CAD build for the part. Positions are in the model's coordinates, mm. A direction names the side the tool comes from. Round coordinates to 2 decimals unless told otherwise and drop trailing zeros. Order: outer loops, then holes, each group sorted by start corner. A loop starts at its lowest first (then second) coordinate and runs counter-clockwise, first axis right, second up. Notation, with made-up numbers: M -30.5,-10 L -0.5,-10 A13 ccw -0.5,8 Z; hole C 69,15 d4. An arc over 180 degrees is marked long. Answer as a JSON object with one key per item and string values. Group by question number.
```python
from build123d import *

# Parameters (mm, degrees)
EXTRUDE_3_DEPTH                 = 15
EXTRUDE_2_DEPTH                 = 1
SKETCH_4_R                      = 5.85
CUT_EXTRUDE_1_DEPTH             = 2
SKIZZE1_W                       = 11.487069154
SKIZZE1_H                       = 62.431572876
SCHNITT_LINEAR_AUSTRAGEN1_DEPTH = 0.5
SKIZZE2_W                       = 1.5
SKIZZE2_H                       = 1.5
AUFSATZ_LINEAR_AUSTRAGEN1_DEPTH = 1.5


with BuildPart() as part:
    # Эскиз1 → Вытянуть-Тонкостенный3 (new body)
    with BuildSketch(Plane.XY):
        Polygon((-21.213203436, -45), (-21.213203436, 45), (0, 66.213203436), (21.213203436, 45), (21.213203436, -45), (0, -66.213203436), align=None)
        Polygon((-20.213203436, -44.585786438), (-20.213203436, 44.585786438), (0, 64.798989873), (20.213203436, 44.585786438), (20.213203436, -44.585786438), (0, -64.798989873), align=None, mode=Mode.SUBTRACT)
    extrude(amount=EXTRUDE_3_DEPTH)

    # Эскиз2 → Бобышка-Вытянуть2 (add)
    with BuildSketch(Plane(origin=(0, 0, 0), x_dir=(-1, 0, 0), z_dir=(0, 0, -1))):
        Polygon((-20.213203436, -44.585786438), (0, -64.798989873), (20.213203436, -44.585786438), (20.213203436, 44.585786438), (0, 64.798989873), (-20.213203436, 44.585786438), align=None)
    extrude(amount=-EXTRUDE_2_DEPTH)

    # Эскиз4 → Вырез-Вытянуть1 (cut)
    with BuildSketch(Plane.XY.offset(1)):
        with Locations((0, 41.215786438)):
            Circle(SKETCH_4_R)
        with Locations((0, -41.215786438)):
            Circle(SKETCH_4_R)
    extrude(amount=-CUT_EXTRUDE_1_DEPTH, mode=Mode.SUBTRACT)

    # Skizze1 → Schnitt-Linear austragen1 (cut)
    with BuildSketch(Plane.XY.offset(1)):
        with Locations((-0.256465423, 0)):
            Rectangle(SKIZZE1_W, SKIZZE1_H)
    extrude(amount=-SCHNITT_LINEAR_AUSTRAGEN1_DEPTH, mode=Mode.SUBTRACT)

    # Skizze2 → Aufsatz-Linear austragen1 (add)
    with BuildSketch(Plane.XY.offset(1)):
        with Locations((6.237069154, 20.465786438)):
            Rectangle(SKIZZE2_W, SKIZZE2_H)
        with Locations((9.237069154, 20.465786438)):
            Rectangle(SKIZZE2_W, SKIZZE2_H)
        with Locations((-6.75, 20.465786438)):
            Rectangle(SKIZZE2_W, SKIZZE2_H)
        with Locations((-9.75, 20.465786438)):
            Rectangle(SKIZZE2_W, SKIZZE2_H)
        with Locations((6.237069154, -20.465786438)):
            Rectangle(SKIZZE2_W, SKIZZE2_H)
        with Locations((9.237069154, -20.465786438)):
            Rectangle(SKIZZE2_W, SKIZZE2_H)
        with Locations((-6.75, -20.465786438)):
            Rectangle(SKIZZE2_W, SKIZZE2_H)
        with Locations((-9.75, -20.465786438)):
            Rectangle(SKIZZE2_W, SKIZZE2_H)
    extrude(amount=AUFSATZ_LINEAR_AUSTRAGEN1_DEPTH)


solid = part.part
```
Item 1: Flat gauge pins, fed straight in: pin 1 Ø8 at (x, y) = (-2.5, 29) entering from -Z; pin 2 Ø8 at (x, y) = (14.5, 30.5) entering from +Z; pin 3 Ø0.6 at (x, z) = (-0.5, 0.5) entering from +Y; pin 4 Ø0.8 at (x, z) = (-9.5, 1.5) entering from -Y. Where does each tip first touch, or does it go through?
Item 2: 3-axis set-ups, long thin cutter, end or side, ignore diameter. For faces 1 (the face through (10, 54.8, 7.9)), 2 (the face through (-0.762, -35.416, 0.507)): which of +Z, -Z, +X, -X, +Y, -Y reach the whole face in a straight line?
Item 3: Drill centre lines: line 1 (Y direction, x = 0, z = 0.3); line 2 (Y direction, x = 0, z = 0.6); line 3 (X direction, y = -29.5, z = 10.5). Where is each one in solid material? Low to high. Write a range as [from, to].
Item 4: Cut at B-B, the plane y = -37.5. Give the cut face in (x, z).
Item 5: Cut at A-A, the plane z = 6. Give the cut face in (x, y).
Item 6: Cut at C-C, the plane x = 13. Give the cut face in (y, z), and give its area (3 significant figures).
Item 7: Cut at D-D, the plane y = -6. Give the cut face in (x, z).
Item 8: Two-plate mould, pull along Y, no slides. Class faces 3 (the face through (10.755, -55.458, 7.395)), 4 (the face through (21.213, 1, 7)), 5 (the face through (-10.2, 54.6, 7.9)): +Y half, -Y half, draft (parallel to the pull), parting line (faces both ways), or undercut.
Response values:
{
 "1": {"pin 1": "z = 0", "pin 2": "z = 1", "pin 3": "y = 66.01", "pin 4": "y = -57.11"},
 "2": {"face 1": "+Z", "face 2": "+Z, -Z"},
 "3": {"line 1": "[-66.21, -47.07], [-35.37, 35.37], [47.07, 66.21]", "line 2": "[-66.21, -47.07], [-35.37, -31.22], [31.22, 35.37], [47.07, 66.21]", "line 3": "[-21.21, -20.21], [20.21, 21.21]"},
 "4": {"outline": "M -21.21,0 L -4.52,0 L -4.52,1 L -20.21,1 L -20.21,15 L -21.21,15 Z; M 4.52,0 L 21.21,0 L 21.21,15 L 20.21,15 L 20.21,1 L 4.52,1 Z"},
 "5": {"outline": "M -21.21,-45 L 0,-66.21 L 21.21,-45 L 21.21,45 L 0,66.21 L -21.21,45 Z; hole M -20.21,-44.59 L 0,-64.8 L 20.21,-44.59 L 20.21,44.59 L 0,64.8 L -20.21,44.59 Z"},
 "6": {"outline": "M -53.21,0 L 53.21,0 L 53.21,15 L 51.8,15 L 51.8,1 L -51.8,1 L -51.8,15 L -53.21,15 Z", "area": "146 mm^2"},
 "7": {"outline": "M -21.21,0 L 21.21,0 L 21.21,15 L 20.21,15 L 20.21,1 L 5.49,1 L 5.49,0.5 L -6,0.5 L -6,1 L -20.21,1 L -20.21,15 L -21.21,15 Z"},
 "8": {"face 3": "-Y half", "face 4": "draft", "face 5": "undercut"}
}
